```python
from build123d import *

# Parameters (mm, degrees)
F1_DEPTH = 60.96
F2_DEPTH = 25.4
F3_R     = 30.6605122421


with BuildPart() as f1:
    # F0 (on Front) → F1 (new body)
    with BuildSketch(Plane.XZ):
        Polygon((24.0515821646, -24.9158906195), (34.4402066399, -3.6266205457), (28.7138756682, 19.3595855869), (9.5520031521, 33.2872264655), (-14.0793577975, 31.6394041346), (-31.1228307591, 15.1871529763), (-33.6035853167, -8.371335846), (-20.3608488424, -28.0127835889), (2.4089550909, -34.5467385632), align=None)
    extrude(amount=F1_DEPTH)

    # F2 (add): a face of the model
    f2_faces = [f1.faces().sort_by_distance(p)[0] for p in [
        (-2.2636773227, -30.48, 32.4633153),
    ]]
    extrude(f2_faces, amount=F2_DEPTH)

    # F3
    f3_edges = [f1.edges().sort_by_distance(p)[0] for p in [
        (-4.030537, -60.96, 57.801788),
    ]]
    fillet(f3_edges, radius=F3_R)


solid = f1.part
```
Verification items for the finished model (mm, model axes). Give positions to 0.01 mm unless a question says otherwise; leave off trailing zeros. Order: outer loops, then holes, each group sorted by start corner. A loop starts at its lowest first (then second) coordinate and runs counter-clockwise, first axis right, second up. Notation, with made-up numbers: (-2.5, -33.75) -> (54.5, -33.75) arc R10 ccw to (54.5, -21.75) -> close; hole circle Ø9 at (16, 64). An arc over 180 degrees is marked (long way). Use a Markdown table: item, result.
1) Section check D-D, the plane y = -34. Record the boundary of the cut face in (x, z), then the cut area to 3 significant figures.
Results:
| item | result |
|---|---|
| outline | (-33.6, -8.37) -> (-20.36, -28.01) -> (2.41, -34.55) -> (24.05, -24.92) -> (34.44, -3.63) -> (28.71, 19.36) -> (9.55, 33.29) -> (7.8, 58.4) -> (-15.83, 56.75) -> (-14.08, 31.64) -> (-31.12, 15.19) -> close |
| area | 4,070 mm² |
2) Section check A-A, the plane y = -15. Record the boundary of the cut face in (x, z), then the cut area to 3 significant figures.
Results:
| item | result |
|---|---|
| outline | (-33.6, -8.37) -> (-20.36, -28.01) -> (2.41, -34.55) -> (24.05, -24.92) -> (34.44, -3.63) -> (28.71, 19.36) -> (9.55, 33.29) -> (7.79, 58.63) -> (-15.85, 56.98) -> (-14.08, 31.64) -> (-31.12, 15.19) -> close |
| area | 4,070 mm² |
3) Section check C-C, the plane x = -25. Record the boundary of the cut face in (y, z), then the cut area to 3 significant figures.
Results:
| item | result |
|---|---|
| outline | (-60.96, -21.13) -> (0, -21.13) -> (0, 21.1) -> (-60.96, 21.1) -> close |
| area | 2,570 mm² |
4) Mould release check, pull along Z, two halves, no side actions. Record for faces 1 (the flat face through (-14.95, -29.83, 44.13)), 2 (the flat face through (8.68, -29.83, 45.78)), 3 (the flat face through (1, -60.96, -4)), 4 (the flat face through (13.08, -30.05, -29.8)): pulls with the +Z half, pulls with the -Z half, needs draft (parallel to the pull), parting line crosses it, or undercut.
Results:
| item | result |
|---|---|
| face 1 | undercut |
| face 2 | pulls with the +Z half |
| face 3 | needs draft |
| face 4 | pulls with the -Z half |
5) Section check B-B, the plane z = 21. Record the boundary of the cut face in (x, y).
Results:
| item | result |
|---|---|
| outline | (-25.1, -60.96) -> (26.46, -60.96) -> (26.46, 0) -> (-25.1, 0) -> close |
6) Material ranges on probe 1 along Y at (x, z) = (-9.5, 27.5); probe 2 along X at (y, z) = (-31, 12); probe 3 along X at (y, z) = (-22.5, 42.5), recorded low to high.
Results:
| item | result |
|---|---|
| probe 1 | -60.95 to 0 |
| probe 2 | -31.46 to 30.55 |
| probe 3 | -14.84 to 8.91 |
7) Depth check by flat-ended pin: pin 1 Ø12 at (y, z) = (-50.5, -17.5) entering from +X; pin 2 Ø1 at (x, y) = (-10.5, -26) entering from -Z; pin 3 Ø1.5 at (x, y) = (-20, -38) entering from +Z; pin 4 Ø5 at (x, z) = (9, 21.5) entering from +Y. Enter the tip coordinate at first touch or a pass-through.
Results:
| item | result |
|---|---|
| pin 1 | x = 30.6 |
| pin 2 | z = -30.99 |
| pin 3 | z = 26.65 |
| pin 4 | y = 0 |
